```python
from build123d import *

# Parameters (mm, degrees)
AUFSATZ_LINEAR_AUSTRAGEN1_DEPTH                      = 400
FASE1_SIZE                                           = 0.5
STIRNSENKUNG_F_R_M3_D_NNKOPF_ZYLINDERSCH_D           = 4
STIRNSENKUNG_F_R_M3_D_NNKOPF_ZYLINDERSCH_CBORE_D     = 6
STIRNSENKUNG_F_R_M3_D_NNKOPF_ZYLINDERSCH_CBORE_DEPTH = 5


with BuildPart() as part:
    # Skizze1 → Aufsatz-Linear austragen1 (new body)
    with BuildSketch(Plane(origin=(0, 0, 0), x_dir=(0, 0, -1), z_dir=(1, 0, 0))):
        with BuildLine():
            Line((6, -4), (-6, -4))
            Line((-6, -4), (-6, 0.25))
            ThreePointArc((-6, 0.25), (-5.25, 1), (-6, 1.75))
            Line((-6, 1.75), (-6, 4))
            Line((-6, 4), (6, 4))
            Line((6, 4), (6, 1.75))
            ThreePointArc((6, 1.75), (5.25, 1), (6, 0.25))
            Line((6, 0.25), (6, -4))
        make_face()
    extrude(amount=AUFSATZ_LINEAR_AUSTRAGEN1_DEPTH)

    # Fase1
    fase1_edges = [part.edges().sort_by_distance(p)[0] for p in [
        (200, 4, 6),
        (200, 4, -6),
    ]]
    chamfer(fase1_edges, length=FASE1_SIZE)

    # Stirnsenkung für M3 Dünnkopf-Zylinderschraube mit Innensechskant1 (through all)
    with Locations(Plane(origin=(12.5, 4, 0), x_dir=(0, 0, 1), z_dir=(0, 1, 0))):
        with Locations((0, 0), (0, 375), (0, 350), (0, 325), (0, 300), (0, 275), (0, 250), (0, 225), (0, 200), (0, 175), (0, 150), (0, 125), (0, 100), (0, 75), (0, 50), (0, 25)):
            CounterBoreHole(STIRNSENKUNG_F_R_M3_D_NNKOPF_ZYLINDERSCH_D / 2, STIRNSENKUNG_F_R_M3_D_NNKOPF_ZYLINDERSCH_CBORE_D / 2, STIRNSENKUNG_F_R_M3_D_NNKOPF_ZYLINDERSCH_CBORE_DEPTH)


solid = part.part
```
Verification items for the finished model (mm, model axes). Coordinates: 2 decimals unless noted, no trailing zeros. Loops run counter-clockwise (first coordinate to the right, second up) from the corner with the lowest first, then second, coordinate; pieces in that order, holes last. Notation, with made-up numbers: (6.25, -40) - (29.25, -40) arc R20 cw to (29.25, -19) - close; hole circle Ø2 at (58, 74.5). An arc over 180 degrees is marked (long way). Put each result on its own line as item: value.
Item 1: Section check A-A (y = -2.5). Give the number of separate pieces and of enclosed holes in the cut face, then the cut area to 3 significant figures.
Conclusion:
separate pieces: 1
enclosed holes: 16
area: 4,600 mm2
Item 2: Section check B-B (x = 77). Enter the section's corners in (y, z).
Conclusion:
outline: (-4, -6) - (0.25, -6) arc R0.75 cw to (1.75, -6) - (3.5, -6) - (4, -5.5) - (4, 5.5) - (3.5, 6) - (1.75, 6) arc R0.75 cw to (0.25, 6) - (-4, 6) - close
Item 3: Scan lines: line 1 along Z through (x, y) = (137.5, 2.45); line 2 along Z through (x, y) = (187.5, -1.55); line 3 along Z through (x, y) = (52, 0.75). Record each from-to range of solid material in increasing order.
Conclusion:
line 1: z = -6 to -3, 3 to 6
line 2: z = -6 to -2, 2 to 6
line 3: z = -5.29 to 5.29
Item 4: Gauge pin test, flat ends, axial feed: pin 1 Ø4.5 at (x, z) = (337.5, 0) entering from -Y; pin 2 Ø4.5 at (x, z) = (237.5, 0) entering from +Y. Record the tip position at first contact, or that the pin passes through.
Conclusion:
pin 1: stops at y = -4
pin 2: stops at y = -1
